Model file for the job. Use its own axes, mm. A direction names the side the tool comes from. Coordinates: 2 decimals unless noted, no trailing zeros. Write each loop counter-clockwise with the first axis right and the second up, starting at its lowest first coordinate (ties: lowest second). Pieces come first, ordered by that corner, then holes. Notation, with made-up numbers: M 81.5,32 L 133.5,32 A22 ccw 133.5,42 Z; hole C 85,52.25 d2. An arc over 180 degrees is marked long. Put each result on its own line as item: value. Start each with the question number.
Q1. Cut at D-D (x = 0). Write the cut outline in (y, z).
Q2. Cut at C-C (y = 49.5). Write the cut outline in (x, z).
Q3. Which spindle directions (+Z, -Z, +X, -X, +Y, -Y) get a long thin tool onto all of the face, cutting with end or side? Do faces 1 (the flat face through (-1, 0, 0)), 2 (the flat face through (0.6, 3, 1)). Say none if no direction does.
Q4. Drop flat-ended pins along their axis: pin 1 (1.1 mm diameter, centred on y = 2.5, z = -1, fed in from -X); pin 2 (1 mm diameter, centred on x = 1.5, y = 21, fed in from -Z); pin 3 (1.1 mm diameter, centred on y = 3, z = -1, fed in from +X). Give the stop position or say it passes through.
Q5. Pull direction Z, two halves, no side cores. Call faces 3 (the flat face through (0, 55.9, 0)), 4 (the cylindrical face through (1, 2, -1)), 5 (the cylindrical face through (-0.766, 27.559, 1.847)): pulls with the +Z half, pulls with the -Z half, needs draft (parallel to the pull), parting line crosses it, or undercut.
Q6. Cut at A-A (y = 2). Write the cut outline in (x, z), then the cut area to 3 significant figures.
Q7. Cut at B-B (z = -0.05). Write the cut outline in (x, y).
Q8. Drill centre lines: line 1 along Y through (x, z) = (-1.2, 0); line 2 along X through (y, z) = (10, 0.6); line 3 along Y through (x, z) = (0.1, -0.7). Where is each one in solid material? Low to high.
```python
from build123d import *

# Parameters (mm, degrees)
SKETCH_1_R               = 2
EXTRUDE_1_DEPTH          = 55.9
CUT_EXTRUDE_1_DEPTH      = 56.97151061
CUT_EXTRUDE_1_DEPTH_BACK = 56.97151061
SKETCH_2_W               = 1.2
SKETCH_2_H               = 10
CUT_EXTRUDE_2_DEPTH      = 56.97151061
CUT_EXTRUDE_2_DEPTH_BACK = 56.97151061
SKETCH_3_R               = 1


with BuildPart() as part:
    # 草图1 → 凸台-拉伸1 (new body)
    with BuildSketch(Plane(origin=(0, 0, 0), x_dir=(1, 0, 0), z_dir=(0, 1, 0))):
        with Locations(Location((0, 0, 0), (0, 0, 270))):
            Circle(SKETCH_1_R)
    extrude(amount=EXTRUDE_1_DEPTH)

    # 草图2 → 切除-拉伸1 (cut, two sides: drawn at the far end of the back side and taken through both)
    with BuildSketch(Plane.XY.offset(-CUT_EXTRUDE_1_DEPTH_BACK)):
        Rectangle(SKETCH_2_W, SKETCH_2_H)
    extrude(amount=CUT_EXTRUDE_1_DEPTH + CUT_EXTRUDE_1_DEPTH_BACK, mode=Mode.SUBTRACT)

    # 草图3 → 切除-拉伸2 (cut, two sides: drawn at the far end of the back side and taken through both)
    with BuildSketch(Plane(origin=(0, 0, 0), x_dir=(0, 0, -1), z_dir=(1, 0, 0)).offset(-CUT_EXTRUDE_2_DEPTH_BACK)):
        with Locations((0, 2)):
            Circle(SKETCH_3_R)
    extrude(amount=CUT_EXTRUDE_2_DEPTH + CUT_EXTRUDE_2_DEPTH_BACK, mode=Mode.SUBTRACT)


solid = part.part
```
Computed values:
1. outline: M 5,-2 L 55.9,-2 L 55.9,2 L 5,2 Z
2. outline: C 0,0 d4
3. face 1: +Z, -Z, +X, -X, -Y
3. face 2: +Z, -Z, -Y
4. pin 1: x = -1.92
4. pin 2: z = -1.73
4. pin 3: x = 1.95
5. face 3: needs draft
5. face 4: undercut
5. face 5: parting line crosses it
6. outline: M -1.73,-1 A2 ccw -0.6,-1.91 L -0.6,-1 Z; M -1.73,1 L -0.6,1 L -0.6,1.91 A2 ccw Z; M 0.6,-1.91 A2 ccw 1.73,-1 L 0.6,-1 Z; M 0.6,1 L 1.73,1 A2 ccw 0.6,1.91 Z
6. area: 2.59 mm2
7. outline: M -2,0 L -0.6,0 L -0.6,1 L -2,1 Z; M -2,3 L -0.6,3 L -0.6,5 L 0.6,5 L 0.6,3 L 2,3 L 2,55.9 L -2,55.9 Z; M 0.6,0 L 2,0 L 2,1 L 0.6,1 Z
8. line 1: 0 to 1, 3 to 55.9
8. line 2: -1.91 to 1.91
8. line 3: 5 to 55.9
